Design review of the part built by this model. Coordinates are the model's own, in mm. A direction names the side the tool comes from. Coordinates: 2 decimals unless noted, no trailing zeros. Loops run counter-clockwise (first coordinate to the right, second up) from the corner with the lowest first, then second, coordinate; pieces in that order, holes last. Notation, with made-up numbers: M 84,56 L 128,56 A24 cw 128,72 Z; hole C 44.5,67 d11. An arc over 180 degrees is marked long. Answer as a JSON object with one key per item and string values. Group by question number.
1. Consider section C-C (z = 124.5). State the section outline as (x, y) points.
2. Consider section B-B (y = 2.5). State the section outline as (x, z) points.
3. Consider section A-A (x = 83.5). State the section outline as (y, z) points.
4. Draft analysis for pull direction Y (two halves, no side actions). For faces 1 (the cylindrical face through (77.04, 18.35, 147.49)), 2 (the cylindrical face through (82.96, 20.48, 53.38)), 3 (the flat face through (68, 16, 52)), state which applies: +Y half, -Y half, draft (parallel to the pull), parting line (faces both ways), or undercut.
5. Consider section D-D (z = 67). State the section outline as (x, y) points.
6. Insertion check: pin 1 (3 mm diameter, centred on x = 65.5, y = 18, fed in from -Z); pin 2 (1.5 mm diameter, centred on x = 78.5, z = 116, fed in from +Y); pin 3 (1 mm diameter, centred on x = 55.5, y = -1.5, fed in from +Z); pin 4 (15.5 mm diameter, centred on y = 3.5, z = 42, fed in from -X). Each pin has a flat end and moves straight along its axis. Give the tip position at first contact, or say it passes through.
7. Machinability: for faces 4 (the flat face through (72.34, 16.07, 99.32)), 5 (the flat face through (80, 8, 33)), 6 (the cylindrical face through (88.465, 2.72, 34.995)), 7 (the flat face through (80, 22.4, 142.9)), which of the approach directions +Z, -Z, +X, -X, +Y, -Y give a long, thin tool a straight path to every point of the face, cutting with its end or side? Answer none if there is none.
8. To check wall thickness, follow probe 1 along X at (y, z) = (10.5, 27); probe 2 along Y at (x, z) = (64.5, 30); probe 3 along X at (y, z) = (11.5, 134). State the ranges of each line that lie inside material, in increasing order.
from build123d import *

# Parameters (mm, degrees)
SKETCH017_R       = 3
EXTRUDE016_DEPTH  = 6
SKETCH016_W       = 23
SKETCH016_H       = 90
EXTRUDE015_DEPTH  = 10
CYLINDER018_R     = 3
CYLINDER018_DEPTH = 25
CYLINDER013_R     = 7
CYLINDER013_DEPTH = 30
CYLINDER012_R     = 10
CYLINDER012_DEPTH = 6
EXTRUDE001_DEPTH  = 6
BOX022_W          = 23
BOX022_H          = 10
BOX022_DEPTH      = 10
CYLINDER021_R     = 2.7
CYLINDER021_DEPTH = 50
CYLINDER020_R     = 5
CYLINDER020_DEPTH = 45


with BuildPart() as union_brazo_central002:
    # Sketch017 → Extrude016 (new body)
    with BuildSketch(Plane(origin=(0, 0, 0), x_dir=(0, -1, 0), z_dir=(-1, 0, 0))):
        with BuildLine():
            ThreePointArc((-10.900695, 145.407872), (-23.024313, 154.355924), (-27.779278, 140.057671))
            Line((-27.779278, 140.057671), (-20.026942, 129.238365))
            Line((-20.026942, 129.238365), (-11.026942, 129.238365))
            Line((-10.900695, 145.407872), (-11.026942, 129.238365))
        make_face()
        with Locations((-19.957954, 144.958669)):
            Circle(SKETCH017_R, mode=Mode.SUBTRACT)
    extrude(amount=EXTRUDE016_DEPTH)


with BuildPart() as union_brazo_central002_1:
    # Extrude016 placement: moved
    add(union_brazo_central002.part.moved(Location((63, 0, 0))))


with BuildPart() as palo_central:
    # Sketch016 → Extrude015 (new body)
    with BuildSketch(Plane.XZ):
        with Locations((68.535034, 86.905613)):
            Rectangle(SKETCH016_W, SKETCH016_H)
        Polygon((68.535034, 64.926588), (61.035034, 51.936207), (76.035034, 51.936207), align=None, mode=Mode.SUBTRACT)
        Polygon((68.535034, 85.416969), (61.035034, 72.426588), (76.035034, 72.426588), align=None, mode=Mode.SUBTRACT)
        Polygon((68.535034, 105.90735), (61.035034, 92.916969), (76.035034, 92.916969), align=None, mode=Mode.SUBTRACT)
        Polygon((68.535034, 126.397731), (61.035034, 113.40735), (76.035034, 113.40735), align=None, mode=Mode.SUBTRACT)
    extrude(amount=EXTRUDE015_DEPTH)


with BuildPart() as palo_central_1:
    # Extrude015 placement: moved
    add(palo_central.part.moved(Location((0, 21, 0))))


with BuildPart() as rotor008:
    # Cylinder018 → Cylinder018 (new body)
    with BuildSketch(Plane(origin=(40, 2.5, 30), x_dir=(0, 0, -1), z_dir=(1, 0, 0))):
        Circle(CYLINDER018_R)
    extrude(amount=CYLINDER018_DEPTH)


with BuildPart() as rotor003:
    # Cylinder013 → Cylinder013 (new body)
    with BuildSketch(Plane(origin=(63, 2.5, 30), x_dir=(0, 0, -1), z_dir=(1, 0, 0))):
        Circle(CYLINDER013_R)
    extrude(amount=CYLINDER013_DEPTH)


with BuildPart() as obj1:
    # Cylinder012 → Cylinder012 (new body)
    with BuildSketch(Plane(origin=(54, 2.5, 30), x_dir=(0, 0, -1), z_dir=(1, 0, 0))):
        Circle(CYLINDER012_R)
    extrude(amount=CYLINDER012_DEPTH)

    # Cut008: cut Rotor003
    add(rotor003.part, mode=Mode.SUBTRACT)

    # Cut011: cut Rotor008
    add(rotor008.part, mode=Mode.SUBTRACT)


with BuildPart() as union_motor_centro:
    # Sketch001 → Extrude001 (new body)
    with BuildSketch(Plane.YZ):
        with BuildLine():
            ThreePointArc((22.654639, 41.99706), (20.679007, 53.483206), (9.335322, 50.808228))
            Line((9.335322, 50.808228), (1.552816, 39.899855))
            ThreePointArc((12.665635, 28.738862), (9.310536, 36.511168), (1.552816, 39.899855))
            Line((22.654639, 41.99706), (12.665635, 28.738862))
        make_face()
    extrude(amount=EXTRUDE001_DEPTH)


with BuildPart() as union_motor_centro_1:
    # Extrude001 placement: moved
    add(union_motor_centro.part.moved(Location((54, -0.35, 0))))

    # Fusion013: union obj1
    add(obj1.part)


with BuildPart() as union_motor_centro001:
    # Link016 base: copy of Union motor centro
    add(union_motor_centro_1.part)


with BuildPart() as union_motor_centro001_1:
    # Link016 placement: moved
    add(union_motor_centro001.part.moved(Location((28.999998, -3e-06, 0))))


with BuildPart() as obj2:
    # Box022 → Box022 (new body)
    with BuildSketch(Plane(origin=(60, 11, 42), x_dir=(1, 0, 0), z_dir=(0, 0, 1))):
        with Locations((11.5, 5)):
            Rectangle(BOX022_W, BOX022_H)
    extrude(amount=BOX022_DEPTH)


with BuildPart() as hueco_rotor:
    # Cylinder021 → Cylinder021 (new body)
    with BuildSketch(Plane(origin=(37, 2.5, 30), x_dir=(0, 0, -1), z_dir=(1, 0, 0))):
        Circle(CYLINDER021_R)
    extrude(amount=CYLINDER021_DEPTH)


with BuildPart() as union_rotor_brazo:
    # Cylinder020 → Cylinder020 (new body)
    with BuildSketch(Plane(origin=(40, 2.5, 30), x_dir=(0, 0, -1), z_dir=(1, 0, 0))):
        Circle(CYLINDER020_R)
    extrude(amount=CYLINDER020_DEPTH)

    # Cut012: cut hueco rotor
    add(hueco_rotor.part, mode=Mode.SUBTRACT)


with BuildPart() as union_rotor_brazo_1:
    # Cut012 placement: moved
    add(union_rotor_brazo.part.moved(Location((9, 0, 0))))

    # Fusion014: union Union motor centro001, Union motor centro, obj2
    add(union_motor_centro001_1.part)
    add(union_motor_centro_1.part)
    add(obj2.part)


with BuildPart() as union_rotor_brazo_2:
    # Fusion014 placement: moved
    add(union_rotor_brazo_1.part.moved(Location((-3, 0, 0))))


with BuildPart() as brazo_central_v2:
    # Link018 base: copy of Union brazo central002
    add(union_brazo_central002_1.part)


with BuildPart() as brazo_central_v2_1:
    # Link018 placement: moved
    add(brazo_central_v2.part.moved(Location((17.000008, -1e-05, 0))))

    # Fusion022: union Union brazo central002, Palo central, Union rotor brazo
    add(union_brazo_central002_1.part)
    add(palo_central_1.part)
    add(union_rotor_brazo_2.part)


solid = brazo_central_v2_1.part
Findings below:
{
 "1": {"outline": "M 57.04,11 L 67.44,11 L 67.44,21 L 57.04,21 Z; M 69.63,11 L 80.04,11 L 80.04,21 L 69.63,21 Z"},
 "2": {"outline": "M 46,25 L 51,25 L 51,20 L 57,20 L 57,25 L 80,25 L 80,20 L 86,20 L 86,25 L 91,25 L 91,27.3 L 46,27.3 Z; M 46,32.7 L 91,32.7 L 91,35 L 86,35 L 86,41.72 L 80,41.72 L 80,35 L 57,35 L 57,41.72 L 51,41.72 L 51,35 L 46,35 Z"},
 "3": {"outline": "M 1.22,39.92 A10 ccw long 12.44,28.9 L 22.3,42 A8 ccw long 8.99,50.81 Z; hole C 2.5,30 d5.4"},
 "4": {"face 1": "undercut", "face 2": "parting line", "face 3": "draft"},
 "5": {"outline": "M 57.04,11 L 80.04,11 L 80.04,21 L 57.04,21 Z"},
 "6": {"pin 1": "stops at z = 41.91", "pin 2": "stops at y = 21", "pin 3": "stops at z = 39.37", "pin 4": "stops at x = 46"},
 "7": {"face 4": "+Y, -Y", "face 5": "none", "face 6": "+X", "face 7": "+Z, +X, +Y, -Y"},
 "8": {"probe 1": "x = 51 to 57, 80 to 86", "probe 2": "y = -2.5 to -0.2, 5.2 to 7.5", "probe 3": "x = 57 to 63, 74 to 80"}
}
